```python
from build123d import *

# Parameters (mm, degrees)
PAD029_DEPTH    = 11.4
SKETCH042_W     = 22.4
SKETCH042_H     = 8.7429971978
PAD030_DEPTH    = 37
SKETCH043_W     = 5
SKETCH043_H     = 5
SKETCH043_R     = 1.4
PAD031_DEPTH    = 1.5
SKETCH044_R     = 2.7
SKETCH044_R_2   = 1.45
SKETCH044_R_3   = 1
POCKET007_DEPTH = 8.75
POCKET010_DEPTH = 11.4
SKETCH055_W     = 20.4
SKETCH055_H     = 35
POCKET011_DEPTH = 7.743
FILLET012_R     = 3.2
FILLET013_R     = 4
SKETCH056_R     = 3
POCKET012_DEPTH = 1
SKETCH057_W     = 6
SKETCH057_H     = 2
POCKET013_DEPTH = 1
PAD040_DEPTH    = 2.65


with BuildPart() as part:
    # Sketch041 → Pad029 (new body)
    with BuildSketch(Plane.XZ):
        with BuildLine():
            ThreePointArc((7, -8.7429971978), (10.0955435713, -4.8497422612), (11.2, 0))
            Line((-11.2, 0), (11.2, 0))
            ThreePointArc((-11.2, 0), (-10.0955435713, -4.8497422612), (-7, -8.7429971978))
            Line((7, -8.7429971978), (-7, -8.7429971978))
        make_face()
    extrude(amount=PAD029_DEPTH)

    # Sketch042 (on Face6 of Pad029) → Pad030 (join)
    with BuildSketch(Plane.XZ.offset(11.4)):
        with Locations((0, -4.3714985989)):
            Rectangle(SKETCH042_W, SKETCH042_H)
    extrude(amount=PAD030_DEPTH)

    # Sketch043 (on Face10 of Pad030) → Pad031 (join)
    with BuildSketch(Plane(origin=(0, 0, 0), x_dir=(-1, 0, 0), z_dir=(0, 0, 1))):
        with Locations((0, 50.9)):
            Rectangle(SKETCH043_W, SKETCH043_H)
        with Locations((0, 50.9)):
            Circle(SKETCH043_R, mode=Mode.SUBTRACT)
    extrude(amount=-PAD031_DEPTH)

    # Sketch044 (on Face15 of Pad031) → Pocket007 (cut)
    with BuildSketch(Plane(origin=(0, 0, 0), x_dir=(-1, 0, 0), z_dir=(0, 0, 1))):
        with Locations((0, 37.1)):
            Circle(SKETCH044_R)
        with Locations((8.7, 16.4)):
            Circle(SKETCH044_R_2)
        with Locations((-8.7, 16.4)):
            Circle(SKETCH044_R_2)
        with Locations((-9.2, 13.4)):
            Circle(SKETCH044_R_3)
        with Locations((9.2, 13.4)):
            Circle(SKETCH044_R_3)
    extrude(amount=-POCKET007_DEPTH, mode=Mode.SUBTRACT)

    # Sketch054 (on Face4 of Pocket007) → Pocket010 (cut)
    with BuildSketch(Plane(origin=(0, 0, 0), x_dir=(1, 0, 0), z_dir=(0, 1, 0))):
        with BuildLine():
            ThreePointArc((-6.6397284881, 7.7429971978), (-9.2672873749, 4.2611482855), (-10.2, 0))
            Line((-10.2, 0), (10.2, 0))
            ThreePointArc((10.2, 0), (9.2672873749, 4.2611482855), (6.6397284881, 7.7429971978))
            Line((-6.6397284881, 7.7429971978), (6.6397284881, 7.7429971978))
        make_face()
    extrude(amount=-POCKET010_DEPTH, mode=Mode.SUBTRACT)

    # Sketch055 (on Face3 of Pocket010) → Pocket011 (cut)
    with BuildSketch(Plane(origin=(0, 0, 0), x_dir=(-1, 0, 0), z_dir=(0, 0, 1))):
        with Locations((0, 29.9)):
            Rectangle(SKETCH055_W, SKETCH055_H)
    extrude(amount=-POCKET011_DEPTH, mode=Mode.SUBTRACT)

    # Fillet012
    fillet012_edges = [part.edges().sort_by_distance(p)[0] for p in [
        (10.2, -47.4, -3.8715),
        (-10.2, -47.4, -3.8715),
    ]]
    fillet(fillet012_edges, radius=FILLET012_R)

    # Fillet013
    fillet013_edges = [part.edges().sort_by_distance(p)[0] for p in [
        (11.2, -48.4, -4.371499),
        (-11.2, -48.4, -4.371499),
    ]]
    fillet(fillet013_edges, radius=FILLET013_R)

    # Sketch056 (on Face10 of Fillet013) → Pocket012 (cut)
    with BuildSketch(Plane(origin=(0, -11.4, 0), x_dir=(1, 0, 0), z_dir=(0, 1, 0))):
        Circle(SKETCH056_R)
    extrude(amount=-POCKET012_DEPTH, mode=Mode.SUBTRACT)

    # Sketch057 (on Face24 of Pocket012) → Pocket013 (cut)
    with BuildSketch(Plane(origin=(0, 0, -8.7429971978), x_dir=(1, 0, 0), z_dir=(0, 0, -1))):
        with Locations((0, 6.5)):
            Rectangle(SKETCH057_W, SKETCH057_H)
    extrude(amount=-POCKET013_DEPTH, mode=Mode.SUBTRACT)

    # Sketch058 → Pad040 (join, symmetric)
    with BuildSketch(Plane.YZ):
        Polygon((-5.5, -8.7429971978), (-5.8, -10.2429971978), (-6.8, -10.2429971978), (-6.8, -11.2429971978), (-5, -11.2429971978), (-4.5, -8.7429971978), align=None)
    extrude(amount=PAD040_DEPTH, both=True)


with BuildPart() as part_1:
    # Body020 placement: moved
    add(part.part.moved(Location((0, 37.1, 0))))


solid = part_1.part
```
Input: part model. Units: mm. Frame: model coordinates. A direction names the side the tool comes from. Coordinates: 2 decimals unless noted, no trailing zeros. Write each loop counter-clockwise with the first axis right and the second up, starting at its lowest first coordinate (ties: lowest second). Pieces come first, ordered by that corner, then holes.
1) Section C-C on y = 20.7. Output: boundary loops of the cut face in (x, z).
2) Section B-B on y = -13.8. Output: boundary loops of the cut face in (x, z), and give its area (3 significant figures).
3) Set-up query: faces 1 (the cylindrical face through (0, 25, -3)), 2 (the flat face through (2.65, 32, -10)), 3 (the flat face through (0, 29.6, -8)), 4 (the flat face through (-10.2, 9, -4)), 5 (the cylindrical face through (9.997, -10.159, -4.31)). Return all of +Z, -Z, +X, -X, +Y, -Y with unobstructed straight access to the full face (end or side cutting, diameter ignored); none if empty.
4) Material intervals for line 1 along Y through (x, z) = (0, -7.95); line 2 along X through (y, z) = (16, -5.75); line 3 along Y through (x, z) = (5.25, -4.25), sorted ascending.
5) Mould query, pull axis Y, two halves, no side actions, for faces 6 (the cylindrical face through (8.74, 24.59, -8.24)), 7 (the flat face through (2.5, -14, -1)), 8 (the cylindrical face through (-10.059, -10.097, -4.31)). Classes: pulls with the +Y half, pulls with the -Y half, needs draft (parallel to the pull), parting line crosses it, or undercut.
6) Section D-D on x = 8.7. Output: boundary loops of the cut face in (y, z).
7) Section A-A on x = 0. State how many separate pieces and enclosed holes the cut face has, and give its area (3 significant figures).
8) Pin query (flat end, axial travel): pin 1 Ø3.5 at (x, y) = (2, 32) entering from +Z; pin 2 Ø1 at (y, z) = (-10, -9) entering from -X; pin 3 Ø2 at (x, z) = (-6.5, -3.5) entering from -Y; pin 4 Ø0.5 at (x, y) = (-9.5, 24.5) entering from +Z. Return the tip coordinate at first contact, or that it passes through.
Check result:
1. outline: (-11.2, -8.74) - (-10.15, -8.74) - (-10.15, -7.74) - (-10.2, -7.74) - (-10.2, 0) - (-11.2, 0) - close; (-7.25, -8.74) - (7.25, -8.74) - (7.25, -7.74) - (-7.25, -7.74) - close; (10.15, -8.74) - (11.2, -8.74) - (11.2, 0) - (10.2, 0) - (10.2, -7.74) - (10.15, -7.74) - close
2. outline: (-2.5, -1.5) - (-1.4, -1.5) - (-1.4, 0) - (-2.5, 0) - close; (1.4, -1.5) - (2.5, -1.5) - (2.5, 0) - (1.4, 0) - close
2. area: 3.30 mm2
3. face 1: +Z, +Y
3. face 2: -Z, +X, +Y, -Y
3. face 3: +Z, -Z
3. face 4: +Z
3. face 5: +Z, -Z, +X, -Y
4. line 1: y = -11.3 to -2.7, 2.7 to 29.6, 31.6 to 37.1
4. line 2: x = -11.2 to -10.2, 10.2 to 11.2
4. line 3: y = -11.3 to -10.3, 24.7 to 25.7
5. face 6: undercut
5. face 7: needs draft
5. face 8: pulls with the -Y half
6. outline: (-11.01, -8.74) - (19.25, -8.74) - (19.25, -7.74) - (-9.81, -7.74) - (-9.81, 0) - (-11.01, 0) - close; (22.15, -8.74) - (22.83, -8.74) - (22.83, -7.74) - (22.15, -7.74) - close; (24.57, -8.74) - (25.7, -8.74) - (25.7, -7.05) - (37.1, -7.05) - (37.1, -5.32) - (25.7, -5.32) - (25.7, 0) - (24.7, 0) - (24.7, -7.74) - (24.57, -7.74) - close
7. separate pieces: 4
7. enclosed holes: 0
7. area: 60.2 mm2
8. pin 1: stops at z = -7.74
8. pin 2: stops at x = -10.49
8. pin 3: stops at y = -11.3
8. pin 4: stops at z = 0
